Autodesk Inventor part; units mm, degrees
ref_plane "YZ Plane" through (0, 0, 0) normal (1, 0, 0) x (0, 1, 0)
ref_plane "XZ Plane" through (0, 0, 0) normal (0, 1, 0) x (-1, 0, 0)
ref_plane "XY Plane" through (0, 0, 0) normal (0, 0, 1) x (1, 0, 0)
sketch "Sketch1" plane through (0, 0, 0) normal (0, 0, 1) x (1, 0, 0)
  line L0 (0, 0) -> (0, 14.3)
  line L1 (115.352, 10) -> (115.352, 9.5)
  line L2 (115.352, 9.5) -> (116.452, 9.5)
  line L3 (116.452, 9.5) -> (116.452, 10)
  line L4 (116.452, 10) -> (131.452, 10)
  line L5 (131.452, 10) -> (131.452, 9.5)
  line L6 (131.452, 9.5) -> (132.552, 9.5)
  line L7 (132.552, 9.5) -> (132.552, 10)
  line L8 (132.552, 10) -> (135.552, 10)
  line L9 (135.552, 10) -> (135.552, 0)
  line L10 (135.552, 0) -> (0, 0)
  line L11 (43, 10) -> (43, 27.75)
  line L12 (43, 27.75) -> (38, 27.75)
  line L13 (0, 14.3) -> (2, 14.3)
  line L14 (2, 14.3) -> (2, 13.8)
  line L15 (2, 13.8) -> (3.1, 13.8)
  line L16 (3.1, 13.8) -> (3.1, 14.3)
  line L17 (3.1, 14.3) -> (38, 14.3)
  line L18 (38, 14.3) -> (38, 27.75)
  line L19 (115.352, 10) -> (100.352, 10)
  line L20 (100.352, 10) -> (100.352, 9.5)
  line L21 (100.352, 9.5) -> (99.252, 9.5)
  line L22 (99.252, 9.5) -> (99.252, 10)
  line L23 (99.252, 10) -> (43, 10)
  dimension "d3" = 1.1
  dimension "d5" = 1.1
  dimension "d6" = 10
  dimension "d8" = 5
  dimension "d9" = 72.352
  dimension "d10" = 27.75
  dimension "d12" = 3
  dimension "d15" = 1.1
  dimension "d16" = 0.5
  dimension "d17" = 2
  dimension "d18" = 34.9
  dimension "d19" = 14.3
  dimension "d20" = 0.5
  dimension "d21" = 0.5
  dimension "d22" = 0.5
  dimension "d23" = 15
  dimension "d39" = 1.1
  dimension "d40" = 0.5
  dimension "d41" = 15
revolve "Revolution1" add sketch "Sketch1" angle 360 about axis through (135.552, 0, 0) along (-1, 0, 0)
sketch "Sketch2" plane through (43, 0, 0) normal (1, 0, 0) x (0, 0, -1)
  arc A0 (19.9153, -3.9332) -> (19.9669, 3.6623) centre (0, 0) ccw
  arc A1 (20.9085, 5.1405) -> (19.9669, 3.6623) centre (21.2333, 3.8946) ccw
  line L0 (20.9085, 5.1405) -> (23.1638, 5.7284)
  arc A2 (24.7533, 4.7239) -> (23.1638, 5.7284) centre (23.4886, 4.4826) ccw
  arc A3 (24.6868, -5.0596) -> (24.7533, 4.7239) centre (0, 0) ccw
  arc A4 (23.0839, -6.0425) -> (24.6868, -5.0596) centre (23.4256, -4.8011) ccw
  line L1 (23.0839, -6.0425) -> (20.8368, -5.424) construction
  arc A5 (19.9153, -3.9332) -> (20.8368, -5.424) centre (21.1784, -4.1826) ccw
  circle A6 centre (20.5409, -12.046) radius 2.1526 construction
  arc A7 (25.2444, 4.8176) -> (23.0377, 6.2122) centre (23.4886, 4.4826) ccw
  line L2 (23.0377, 6.2122) -> (20.7824, 5.6243)
  arc A8 (20.7824, 5.6243) -> (19.4751, 3.5721) centre (21.2333, 3.8946) ccw
  arc A9 (19.4248, -3.8363) -> (19.4751, 3.5721) centre (0, 0) ccw
  arc A10 (19.4248, -3.8363) -> (20.7041, -5.906) centre (21.1784, -4.1826) ccw
  line L3 (20.7041, -5.906) -> (22.9512, -6.5245)
  arc A11 (22.9512, -6.5245) -> (25.1767, -5.16) centre (23.4256, -4.8011) ccw
  arc A12 (25.1767, -5.16) -> (25.2444, 4.8176) centre (0, 0) ccw
  circle A13 centre (20.5409, -12.046) radius 2.6526
  arc A14 (17.126, 16.6141) -> (17.057, 19.2236) centre (15.8707, 17.8866) ccw
  line L4 (15.4668, 14.9772) -> (17.126, 16.6141)
  arc A15 (13.0347, 14.9042) -> (15.4668, 14.9772) centre (14.2115, 16.2497) ccw
  arc A16 (13.0347, 14.9042) -> (6.644, 18.652) centre (0, 0) ccw
  arc A17 (5.5204, 20.8102) -> (6.644, 18.652) centre (7.2438, 20.3359) ccw
  line L5 (6.1389, 23.0574) -> (5.5204, 20.8102)
  arc A18 (8.45, 24.2711) -> (6.1389, 23.0574) centre (7.8623, 22.583) ccw
  arc A19 (17.057, 19.2236) -> (8.45, 24.2711) centre (0, 0) ccw
  circle A20 centre (20.7026, 11.7659) radius 2.6526
  arc A21 (-5.8252, 23.1386) -> (-8.1196, 24.3836) centre (-7.5549, 22.6877) ccw
  line L6 (-5.2373, 20.8833) -> (-5.8252, 23.1386)
  arc A22 (-6.3901, 18.7405) -> (-5.2373, 20.8833) centre (-6.967, 20.4324) ccw
  arc A23 (-6.3901, 18.7405) -> (-12.8311, 15.0799) centre (0, 0) ccw
  arc A24 (-15.262, 15.1859) -> (-12.8311, 15.0799) centre (-13.9895, 16.4412) ccw
  line L7 (-16.8988, 16.8451) -> (-15.262, 15.1859)
  arc A25 (-16.7944, 19.4535) -> (-16.8988, 16.8451) centre (-15.6263, 18.1004) ccw
  arc A26 (-8.1196, 24.3836) -> (-16.7944, 19.4535) centre (0, 0) ccw
  circle A27 centre (0.1617, 23.812) radius 2.6526
  arc A28 (-22.9512, 6.5245) -> (-25.1767, 5.16) centre (-23.4256, 4.8011) ccw
  line L8 (-20.7041, 5.906) -> (-22.9512, 6.5245)
  arc A29 (-19.4248, 3.8363) -> (-20.7041, 5.906) centre (-21.1784, 4.1826) ccw
  arc A30 (-19.4248, 3.8363) -> (-19.4751, -3.5721) centre (0, 0) ccw
  arc A31 (-20.7824, -5.6243) -> (-19.4751, -3.5721) centre (-21.2333, -3.8946) ccw
  line L9 (-23.0377, -6.2122) -> (-20.7824, -5.6243)
  arc A32 (-25.2444, -4.8176) -> (-23.0377, -6.2122) centre (-23.4886, -4.4826) ccw
  arc A33 (-25.1767, 5.16) -> (-25.2444, -4.8176) centre (0, 0) ccw
  circle A34 centre (-20.5409, 12.046) radius 2.6526
  arc A35 (-17.126, -16.6141) -> (-17.057, -19.2236) centre (-15.8707, -17.8866) ccw
  line L10 (-15.4668, -14.9772) -> (-17.126, -16.6141)
  arc A36 (-13.0347, -14.9042) -> (-15.4668, -14.9772) centre (-14.2115, -16.2497) ccw
  arc A37 (-13.0347, -14.9042) -> (-6.644, -18.652) centre (0, 0) ccw
  arc A38 (-5.5204, -20.8102) -> (-6.644, -18.652) centre (-7.2438, -20.3359) ccw
  line L11 (-6.1389, -23.0574) -> (-5.5204, -20.8102)
  arc A39 (-8.45, -24.2711) -> (-6.1389, -23.0574) centre (-7.8623, -22.583) ccw
  arc A40 (-17.057, -19.2236) -> (-8.45, -24.2711) centre (0, 0) ccw
  circle A41 centre (-20.7026, -11.7659) radius 2.6526
  arc A42 (5.8252, -23.1386) -> (8.1196, -24.3836) centre (7.5549, -22.6877) ccw
  line L12 (5.2373, -20.8833) -> (5.8252, -23.1386)
  arc A43 (6.3901, -18.7405) -> (5.2373, -20.8833) centre (6.967, -20.4324) ccw
  arc A44 (6.3901, -18.7405) -> (12.8311, -15.0799) centre (0, 0) ccw
  arc A45 (15.262, -15.1859) -> (12.8311, -15.0799) centre (13.9895, -16.4412) ccw
  line L13 (16.8988, -16.8451) -> (15.262, -15.1859)
  arc A46 (16.7944, -19.4535) -> (16.8988, -16.8451) centre (15.6263, -18.1004) ccw
  arc A47 (8.1196, -24.3836) -> (16.7944, -19.4535) centre (0, 0) ccw
  circle A48 centre (-0.1617, -23.812) radius 2.6526
  point P0 (0, 0)
  dimension "d24" = 0.5
  dimension "d25" = 0.5
  dimension "d28" = 360
extrude "Extrusion1" cut sketch "Sketch2" against normal through all
sketch "Sketch3" plane through (0, 0, 0) normal (-1, 0, 0) x (0, 0, 1)
  circle A0 centre (0, 0) radius 14.3
  point P0 (0, 0)
  point P1 (0, 0)
hole "Hole1" at (0, 0, 0) direction (1, 0, 0) diameter 15 depth 38
properties part number "Center Axle" material "Steel, Mild"
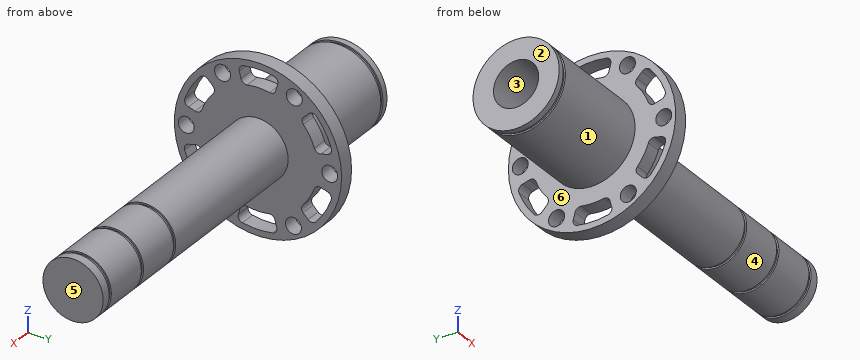
Read the model definition and answer for the solid it produces. Units are mm, in the model's axes. Face numbers are marked on the shaded views. A direction names the side the tool comes from. Give positions to 0.01 mm unless a question says otherwise; leave off trailing zeros. Write each loop counter-clockwise with the first axis right and the second up, starting at its lowest first coordinate (ties: lowest second). Pieces come first, ordered by that corner, then holes. Notation, with made-up numbers: (80, 24.25) - (99, 24.25) arc R35 cw to (99, 56.25) - close; hole circle Ø8 at (28, 65.25). An arc over 180 degrees is marked (long way). Use CSV: the item, a comma, the result in double quotes. Start each with the question number.
Item 1: The mould has two halves that part along Y. Classify the marked faces 1, 2 and 3: pulls with the +Y half, pulls with the -Y half, needs draft (parallel to the pull), parting line crosses it, or undercut.
Item 2: Flat-ended cylindrical pins translate along their axes: P1, Ø4, axis at y = -12.05, z = -20.54, coming from the +X side (1 decimal); P2, Ø2, axis at x = 96.5, z = -2, coming from the +Y side; P3, Ø7, axis at y = 12.05, z = 20.54, coming from the +X side; P4, Ø5, axis at x = 63, z = 7, coming from the +Y side. Find the tip coordinate at first contact, or state that the pin passes through.
Item 3: The part is cut by section D-D, the plane x = 65. Give the vertices of the cut face in (y, z).
Item 4: The part is cut by section B-B, the plane y = 0. Count the separate pieces of the cut face and the enclosed holes in it, and give its area (3 significant figures).
Item 5: For the marked faces 4, 5 and 6, determine the directions among +Z, -Z, +X, -X, +Y, -Y from which every point of the face is accessible in a straight line to the end or side of a thin tool.
Item 6: The part is cut by section A-A, the plane x = 15. Give the vertices of the cut face in (y, z).
Item 7: Consider line 1 (Y direction, x = 22.5, z = 0.5); line 2 (X direction, y = -19.5, z = -3); line 3 (X direction, y = -6.5, z = -2). Determine where each line is inside the solid, lowest interval first.
Taken from the geometry:
1,face 1,"parting line crosses it"
1,face 2,"needs draft"
1,face 3,"undercut"
2,P1,"through"
2,P2,"y = 9.95"
2,P3,"x = 43"
2,P4,"y = 8.93"
3,outline,"circle Ø20 at (0, 0)"
4,separate pieces,"3"
4,enclosed holes,"0"
4,area,"2,580 mm2"
5,face 4,"+X"
5,face 5,"+Z, -Z, +X, +Y, -Y"
5,face 6,"-X"
6,outline,"circle Ø28.6 at (0, 0); hole circle Ø15 at (0, 0)"
7,line 1,"-14.29 to -7.48, 7.48 to 14.29"
7,line 2,"38 to 43"
7,line 3,"38 to 135.55"
